The model under review builds one solid part; all positions refer to its coordinate system, in mm. A direction names the side the tool comes from. Give positions to 0.01 mm unless a question says otherwise; leave off trailing zeros. Loops run counter-clockwise (first coordinate to the right, second up) from the corner with the lowest first, then second, coordinate; pieces in that order, holes last. Notation, with made-up numbers: M -32,4.25 L -24,4.25 A19 ccw -24,22.25 Z; hole C 60.5,32.5 d6. An arc over 180 degrees is marked long. One line per item, written item: value. Start each with the question number.
Q1. We need section A-A on y = -13. Write out the cut boundary in (x, z).
Q2. To check wall thickness, follow line 1 along X through (y, z) = (-3, 44); line 2 along Z through (x, y) = (12.7, -11); line 3 along Y through (x, z) = (68.5, 11). State the ranges of each line that lie inside material, in increasing order. Write a range as from..to.
Q3. We need section C-C on z = 28.5. Write out the cut boundary in (x, y), plus the area to 3 significant figures.
Q4. Mouldability with a two-part tool opening along Y and no side actions: class faces 6 (the face through (73.448, -7.889, 18.904)), 7 (the face through (51, -45.974, 8)), 8 (the face through (51, -38.1, 8)) as released by +Y, released by -Y, zero draft, split by the parting line, or undercut.
Q5. We need section B-B on z = 6. Write out the cut boundary in (x, y).
Q6. For pin 1 (5 mm diameter, centred on x = 54.5, y = -40.5, fed in from +Z), flat-tipped, find the tip position at first contact; note if it passes through.
Q7. We need section D-D on x = 88.9. Write out the cut boundary in (y, z), plus the area to 3 significant figures.
Q8. For faces 1 (the face through (25.4, -31.6, 8.1)), 2 (the face through (13, -20.7, 8.1)), 3 (the face through (11.873, -7.889, 50.746)), 4 (the face through (76.2, -8, 35)), 5 (the face through (50, -23, 16.002)), list the 3-axis set-ups (+Z, -Z, +X, -X, +Y, -Y) from which the entire face can be reached by the end or side of a thin tool; tool diameter is ignored.
```python
from build123d import *

# Parameters (mm, degrees)
F0_R     = 6.35
F1_DEPTH = 16.002
F2_W     = 101.6
F2_H     = 16.002
F3_DEPTH = 50.8
F5_DEPTH = 16.003


with BuildPart() as f1:
    # F0 (on Front) → F1 (new body)
    with BuildSketch(Plane.XZ):
        with BuildLine():
            Line((101.6, 0), (101.6, 44.45))
            ThreePointArc((101.6, 44.45), (88.9, 57.15), (76.2, 44.45))
            Line((76.2, 44.45), (76.2, 25.654))
            ThreePointArc((76.2, 25.654), (73.372995, 18.829005), (66.548, 16.002))
            Line((66.548, 16.002), (35.052, 16.002))
            ThreePointArc((35.052, 16.002), (28.227005, 18.829005), (25.4, 25.654))
            Line((25.4, 25.654), (25.4, 44.45))
            ThreePointArc((25.4, 44.45), (12.7, 57.15), (0, 44.45))
            Line((0, 44.45), (0, 0))
            Line((0, 0), (101.6, 0))
        make_face()
        with Locations((12.7, 44.45)):
            Circle(F0_R, mode=Mode.SUBTRACT)
        with Locations((88.9, 44.45)):
            Circle(F0_R, mode=Mode.SUBTRACT)
    extrude(amount=F1_DEPTH)

    # F2 (on face) → F3 (join)
    with BuildSketch(Plane.XZ.offset(16.002)):
        with Locations((50.8, 8.001)):
            Rectangle(F2_W, F2_H)
    extrude(amount=F3_DEPTH)

    # F4 (on face) → F5 (cut, through all)
    with BuildSketch(Plane.XY.offset(16.002)):
        with BuildLine():
            ThreePointArc((31.75, -45.974), (21.692113, -41.807887), (17.526, -31.75))
            ThreePointArc((17.526, -31.75), (12.913518, -20.614482), (1.778, -16.002))
            Line((1.778, -16.002), (0, -16.002))
            Line((0, -16.002), (0, -66.802))
            Line((0, -66.802), (101.6, -66.802))
            Line((101.6, -66.802), (101.6, -16.002))
            Line((101.6, -16.002), (99.822, -16.002))
            ThreePointArc((99.822, -16.002), (88.686482, -20.614482), (84.074, -31.75))
            ThreePointArc((84.074, -31.75), (79.907887, -41.807887), (69.85, -45.974))
            Line((69.85, -45.974), (31.75, -45.974))
        make_face()
        with BuildLine():
            Line((69.85, -25.4), (31.75, -25.4))
            ThreePointArc((31.75, -25.4), (25.4, -31.75), (31.75, -38.1))
            Line((31.75, -38.1), (69.85, -38.1))
            ThreePointArc((69.85, -38.1), (76.2, -31.75), (69.85, -25.4))
        make_face()
    extrude(amount=-F5_DEPTH, mode=Mode.SUBTRACT)


solid = f1.part
```
Solved:
1. outline: M 0,0 L 101.6,0 L 101.6,44.45 A12.7 ccw 76.2,44.45 L 76.2,25.65 A9.65 cw 66.55,16 L 35.05,16 A9.65 cw 25.4,25.65 L 25.4,44.45 A12.7 ccw 0,44.45 Z; hole C 12.7,44.45 d12.7; hole C 88.9,44.45 d12.7
2. line 1: 0..6.37, 19.03..25.4, 76.2..82.57, 95.23..101.6
2. line 2: 0..38.1, 50.8..57.15
2. line 3: -45.97..-38.1, -25.4..0
3. outline: M 0,-16 L 25.4,-16 L 25.4,0 L 0,0 Z; M 76.2,-16 L 101.6,-16 L 101.6,0 L 76.2,0 Z
3. area: 813 mm2
4. face 6: zero draft
4. face 7: released by -Y
4. face 8: undercut
5. outline: M 0,-16 L 1.78,-16 A15.75 cw 17.53,-31.75 A14.22 ccw 31.75,-45.97 L 69.85,-45.97 A14.22 ccw 84.07,-31.75 A15.75 cw 99.82,-16 L 101.6,-16 L 101.6,0 L 0,0 Z; hole M 31.75,-38.1 L 69.85,-38.1 A6.35 ccw 69.85,-25.4 L 31.75,-25.4 A6.35 ccw Z
6. pin 1: z = 16
7. outline: M -20.4,0 L 0,0 L 0,38.1 L -16,38.1 L -16,16 L -20.4,16 Z; M -16,50.8 L 0,50.8 L 0,57.15 L -16,57.15 Z
7. area: 782 mm2
8. face 1: +Z, -Z
8. face 2: +Z, -Z, -X, -Y
8. face 3: +Y, -Y
8. face 4: +Z, +Y, -Y
8. face 5: +Z, -Y
